```python
from build123d import *

# Parameters (mm, degrees)
F3_D     = 5
F3_DEPTH = 2
F3_TIP   = 1.5021515476


with BuildPart() as f1:
    # F0 (on Top) → F1 (revolve)
    with BuildSketch(Plane.XY):
        with BuildLine():
            Line((-28, 0), (-35, 0))
            Line((-35, 0), (-35, -1.5))
            Line((-35, -1.5), (-30, -6))
            Line((-30, -6), (0, -6))
            Line((0, -6), (0, -4))
            Line((0, -4), (-27.5, -4))
            ThreePointArc((-27.5, -4), (-27.8535533906, -3.8535533906), (-28, -3.5))
            Line((-28, -3.5), (-28, 0))
        make_face()
    revolve(axis=Axis((0, -2.242507413, 0), (0, -1, 0)))

    # F3
    with Locations(Plane(origin=(0, 0, 0), x_dir=(1, 0, 0), z_dir=(0, 1, 0))):
        with Locations((0, -31.5), (29.9582802633, -9.7340353228), (18.5152354472, 25.4840353228), (-18.5152354472, 25.4840353228), (-29.9582802633, -9.7340353228)):
            Hole(F3_D / 2, depth=F3_DEPTH)
            with Locations((0, 0, -(F3_DEPTH + F3_TIP / 2))):  # 118° drill point
                Cone(0, F3_D / 2, F3_TIP, mode=Mode.SUBTRACT)


solid = f1.part
```
Here's how the part is built. I have some questions about the finished solid (model axes, mm). A direction names the side the tool comes from. Round coordinates to 2 decimals unless told otherwise and drop trailing zeros. Order: outer loops, then holes, each group sorted by start corner. A loop starts at its lowest first (then second) coordinate and runs counter-clockwise, first axis right, second up. Notation, with made-up numbers: M -9,31 L 26,31 A6 cw 26,42 Z; hole C 64.25,40 d10. An arc over 180 degrees is marked long. Answer in a Markdown table with one row per item.
Item 1: For faces 1 (the face through (0, -4, 0)), 2 (the face through (28, -1, 21)), which set-ups out of +Z, -Z, +X, -X, +Y, -Y let a thin tool reach every point of the face, with its end or its side?
A:
| item | result |
|---|---|
| face 1 | +Y |
| face 2 | +Y, -Y |
Item 2: I'm going to push flat-ended pins straight in: pin 1 (1.5 mm diameter, centred on x = 0.5, y = -4, fed in from -Z); pin 2 (1.5 mm diameter, centred on x = -2, y = -3.5, fed in from +Z); pin 3 (3 mm diameter, centred on x = -9.5, z = 6.5, fed in from +Y). Where does each tip first touch, or does it pass through?
A:
| item | result |
|---|---|
| pin 1 | stops at z = -33.05 |
| pin 2 | stops at z = 33.55 |
| pin 3 | stops at y = -4 |
Item 3: Imagine slicing it at A-A, the plane z = 0. Write out the boundary of the cut face in (x, y), and give its area (3 significant figures).
A:
| item | result |
|---|---|
| outline | M -35,-1.5 L -30,-6 L 30,-6 L 35,-1.5 L 35,0 L 28,0 L 28,-3.5 A0.5 cw 27.5,-4 L -27.5,-4 A0.5 cw -28,-3.5 L -28,0 L -35,0 Z |
| area | 174 mm2 |
Item 4: Imagine slicing it at B-B, the plane y = -5.2. Write out the boundary of the cut face in (x, z).
A:
| item | result |
|---|---|
| outline | C 0,0 d61.78 |
Item 5: If I drill on L1, parallel to Z at x = 0, y = -0.75; L2, parallel to X at y = -1.15, z = 0; L3, parallel to Z at x = -2, y = -0.8, over which ranges is the centre line in solid material (lowest first)? Write a range as from..to.
A:
| item | result |
|---|---|
| L1 | z = -35..-28, 28..29, 34..35 |
| L2 | x = -35..-28, 28..35 |
| L3 | z = -34.94..-27.93, 27.93..30, 33..34.94 |
Item 6: Thinking about a two-plate mould opening in Z: for faces 3 (the face through (-19.86, -1.01, -27.59)), 4 (the face through (-18.86, -3.24, -25.22)), 5 (the face through (24, -5.78, 18.4)), 6 (the face through (-0.2, 0, 28.4)), which applies, +Z half, -Z half, draft (parallel to the pull), parting line (faces both ways), or undercut?
A:
| item | result |
|---|---|
| face 3 | undercut |
| face 4 | undercut |
| face 5 | parting line |
| face 6 | draft |
